CAD build for the part. Positions are in the model's coordinates, mm. Face numbers are marked on the shaded views. Coordinates: 2 decimals unless noted, no trailing zeros. Loops run counter-clockwise (first coordinate to the right, second up) from the corner with the lowest first, then second, coordinate; pieces in that order, holes last. Notation, with made-up numbers: (82, 23) - (122, 23) arc R16 cw to (122, 44) - close; hole circle Ø1 at (15.25, -3). An arc over 180 degrees is marked (long way). Put each result on its own line as item: value.
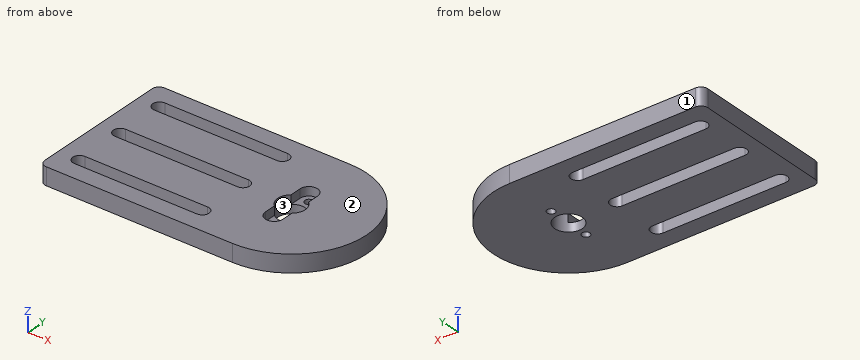
```python
from build123d import *

# Parameters (mm, degrees)
SKETCH1_R           = 5
SKETCH1_R_2         = 1.45
BOSS_EXTRUDE1_DEPTH = 6.35
FILLET1_R           = 2.54
FILLET2_R           = 2.54
CUT_EXTRUDE1_DEPTH  = 3.175


with BuildPart() as part:
    # Sketch1 → Boss-Extrude1 (new body)
    with BuildSketch(Plane.XY):
        with BuildLine():
            Line((-4.497024954, -27.626960595), (-4.497024954, 26.828916206))
            Line((-4.497024954, 26.828916206), (65.352975046, 26.828916206))
            ThreePointArc((65.352975046, 26.828916206), (92.580913446, -0.399022195), (65.352975046, -27.626960595))
            Line((65.352975046, -27.626960595), (-4.497024954, -27.626960595))
        make_face()
        with Locations((65.352975046, -0.399022195)):
            Circle(SKETCH1_R, mode=Mode.SUBTRACT)
        with Locations((65.352975046, 7.600977805)):
            Circle(SKETCH1_R_2, mode=Mode.SUBTRACT)
        with Locations((65.352975046, -8.399022195)):
            Circle(SKETCH1_R_2, mode=Mode.SUBTRACT)
        with BuildLine():
            Line((47.572975046, 15.608916206), (3.122975046, 15.608916206))
            ThreePointArc((3.122975046, 15.608916206), (0.687975046, 18.043916206), (3.122975046, 20.478916206))
            Line((3.122975046, 20.478916206), (47.572975046, 20.478916206))
            ThreePointArc((47.572975046, 20.478916206), (50.007975046, 18.043916206), (47.572975046, 15.608916206))
        make_face(mode=Mode.SUBTRACT)
        with BuildLine():
            Line((3.122975046, 2.348787201), (47.572975046, 2.348787201))
            ThreePointArc((47.572975046, 2.348787201), (50.007975046, -0.086212799), (47.572975046, -2.521212799))
            Line((47.572975046, -2.521212799), (3.122975046, -2.521212799))
            ThreePointArc((3.122975046, -2.521212799), (0.687975046, -0.086212799), (3.122975046, 2.348787201))
        make_face(mode=Mode.SUBTRACT)
        with BuildLine():
            Line((3.122975046, -16.406960595), (47.572975046, -16.406960595))
            ThreePointArc((47.572975046, -16.406960595), (50.007975046, -18.841960595), (47.572975046, -21.276960595))
            Line((47.572975046, -21.276960595), (3.122975046, -21.276960595))
            ThreePointArc((3.122975046, -21.276960595), (0.687975046, -18.841960595), (3.122975046, -16.406960595))
        make_face(mode=Mode.SUBTRACT)
    extrude(amount=BOSS_EXTRUDE1_DEPTH)

    # Fillet1
    fillet1_edges = [part.edges().sort_by_distance(p)[0] for p in [
        (-4.497024954, -27.626960595, 3.175),
    ]]
    fillet(fillet1_edges, radius=FILLET1_R)

    # Fillet2
    fillet2_edges = [part.edges().sort_by_distance(p)[0] for p in [
        (-4.497024954, 26.828916206, 3.175),
    ]]
    fillet(fillet2_edges, radius=FILLET2_R)

    # Sketch2 → Cut-Extrude1 (cut)
    with BuildSketch(Plane.XY.offset(6.35)):
        with BuildLine():
            Line((68.527975046, 7.600977805), (68.527975046, -8.399022195))
            ThreePointArc((68.527975046, -8.399022195), (65.352975046, -11.574022195), (62.177975046, -8.399022195))
            Line((62.177975046, -8.399022195), (62.177975046, 7.600977805))
            ThreePointArc((62.177975046, 7.600977805), (65.352975046, 10.775977805), (68.527975046, 7.600977805))
        make_face()
    extrude(amount=-CUT_EXTRUDE1_DEPTH, mode=Mode.SUBTRACT)


solid = part.part
```
Q1. Slice it at C-C, the plane y = 0.5. Give the cut face in (x, z), then the cut area to 3 significant figures.
Determined:
outline: (-4.5, 0) - (0.76, 0) - (0.76, 6.35) - (-4.5, 6.35) - close; (49.94, 0) - (60.43, 0) - (60.43, 6.35) - (49.94, 6.35) - close; (70.27, 0) - (92.57, 0) - (92.57, 6.35) - (70.27, 6.35) - close
area: 242 mm2
Q2. Slice it at A-A, the plane x = 37. Give the cut face in (y, z), then the cut area to 3 significant figures.
Determined:
outline: (-27.63, 0) - (-21.28, 0) - (-21.28, 6.35) - (-27.63, 6.35) - close; (-16.41, 0) - (-2.52, 0) - (-2.52, 6.35) - (-16.41, 6.35) - close; (2.35, 0) - (15.61, 0) - (15.61, 6.35) - (2.35, 6.35) - close; (20.48, 0) - (26.83, 0) - (26.83, 6.35) - (20.48, 6.35) - close
area: 253 mm2
Q3. Mould opens along Y. For the marked faces 1, 2 and 3 say: +Y half, -Y half, draft (parallel to the pull), parting line (faces both ways), or undercut.
Determined:
face 1: +Y half
face 2: draft
face 3: undercut
Q4. Slice it at D-D, the plane x = 73. Give the cut face in (y, z), then the cut area to 3 significant figures.
Determined:
outline: (-26.53, 0) - (25.73, 0) - (25.73, 6.35) - (-26.53, 6.35) - close
area: 332 mm2
Q5. Wall check: L1, parallel to Y at x = 18, z = 1.5; L2, parallel to Y at x = 48, z = 0.5; L3, parallel to X at y = 18, z = 2.5. Give the ranges that are in metal, low to high. Write a range as from..to.
Determined:
L1: -27.63..-21.28, -16.41..-2.52, 2.35..15.61, 20.48..26.83
L2: -27.63..-21.24, -16.44..-2.48, 2.31..15.65, 20.44..26.83
L3: -4.5..0.69, 50.01..85.42
Q6. Slice it at B-B, the plane z = 4.75. Give the cut face in (x, y) (3 decimals), then the cut area to 3 significant figures.
Determined:
outline: (-4.497, -25.087) arc R2.54 ccw to (-1.957, -27.627) - (65.353, -27.627) arc R27.228 ccw to (65.353, 26.829) - (-1.957, 26.829) arc R2.54 ccw to (-4.497, 24.289) - close; hole (3.123, -21.277) - (47.573, -21.277) arc R2.435 ccw to (47.573, -16.407) - (3.123, -16.407) arc R2.435 ccw to start; hole (3.123, -2.521) - (47.573, -2.521) arc R2.435 ccw to (47.573, 2.349) - (3.123, 2.349) arc R2.435 ccw to start; hole (3.123, 15.609) - (47.573, 15.609) arc R2.435 ccw to (47.573, 20.479) - (3.123, 20.479) arc R2.435 ccw to start; hole (62.178, -8.399) arc R3.175 ccw to (68.528, -8.399) - (68.528, -4.262) arc R5 ccw to (68.528, 3.464) - (68.528, 7.601) arc R3.175 ccw to (62.178, 7.601) - (62.178, 3.464) arc R5 ccw to (62.178, -4.262) - close
area: 4,110 mm2
Q7. Pin check, flat tips, straight feed: pin 1 Ø1 at (y, z) = (6, 4.5) entering from +X; pin 2 Ø1 at (y, z) = (-6, 5.5) entering from +X; pin 3 Ø1 at (x, z) = (71.5, 5) entering from +Y. Stop position of each tip, or through.
Determined:
pin 1: x = 91.93
pin 2: x = 92.1
pin 3: y = 26.24
